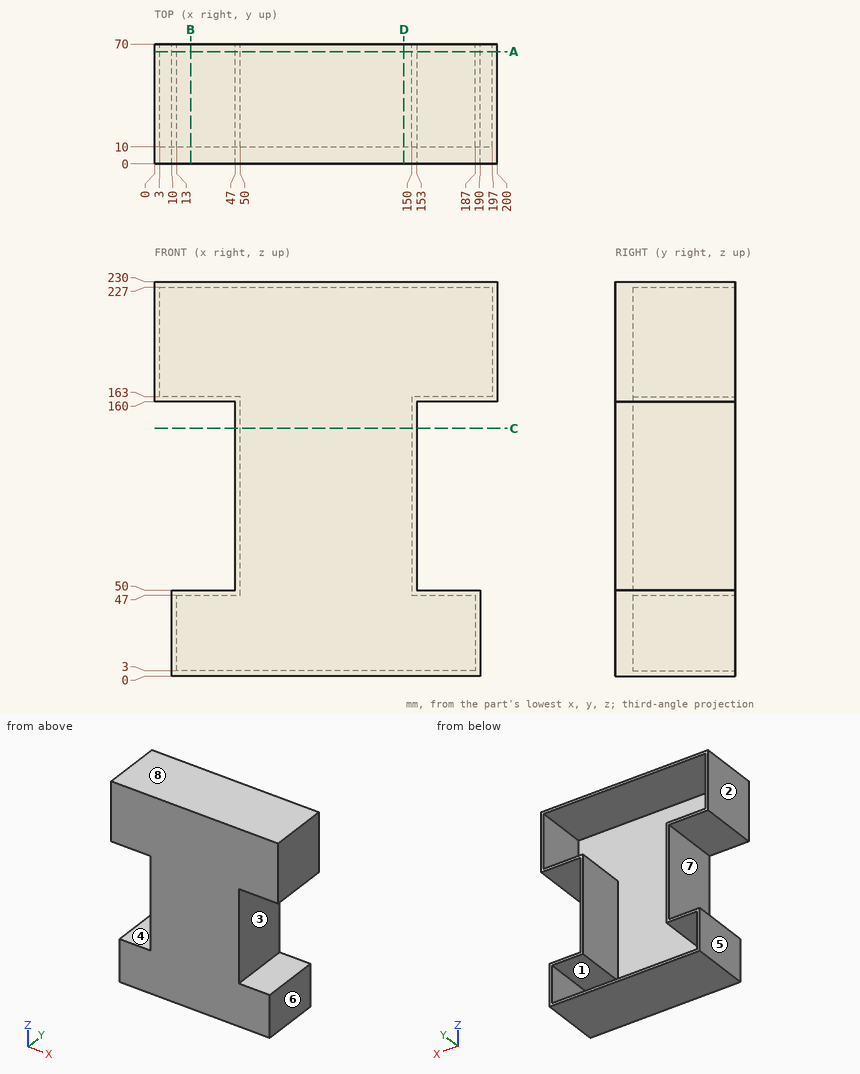
Geometry: see drawing. Coordinates: mm, zero at the bounding-box minimum. A direction names the side the tool comes from. Coordinates: 2 decimals unless noted, no trailing zeros. Loops run counter-clockwise (first coordinate to the right, second up) from the corner with the lowest first, then second, coordinate; pieces in that order, holes last. Notation, with made-up numbers: (-26.75, -22.5) - (6.25, -22.5) arc R24 cw to (6.25, -11.5) - close; hole circle Ø7 at (-7.5, 76). An arc over 180 degrees is marked (long way). Answer in a Markdown table with one row per item.
(1) Cut plane C-C on z = 144.5. Output: boundary loops of the cut face in (x, y), plus the area to 3 significant figures.
Model answer:
| item | result |
|---|---|
| outline | (47, 0) - (153, 0) - (153, 70) - (150, 70) - (150, 10) - (50, 10) - (50, 70) - (47, 70) - close |
| area | 1,420 mm² |
(2) Pin query (flat end, axial travel): P1, Ø1.5, axis at y = 41, z = 149, coming from the -X side; P2, Ø4, axis at x = 52.5, z = 33.5, coming from the +Y side; P3, Ø12, axis at y = 59, z = 34.5, coming from the +X side. Return the tip coordinate at first contact, or that it passes through.
Model answer:
| item | result |
|---|---|
| P1 | stops at x = 47 |
| P2 | stops at y = 10 |
| P3 | stops at x = 190 |
(3) Material intervals for L1, parallel to Z at x = 36, y = 66; L2, parallel to Z at x = 64, y = 55.5; L3, parallel to X at y = 18, z = 167.5, sorted ascending. Write a range as from..to.
Model answer:
| item | result |
|---|---|
| L1 | z = 0..3, 47..50, 160..163, 227..230 |
| L2 | z = 0..3, 227..230 |
| L3 | x = 0..3, 197..200 |
(4) Cut plane B-B on x = 21. Output: boundary loops of the cut face in (y, z), plus the area to 3 significant figures.
Model answer:
| item | result |
|---|---|
| outline | (0, 0) - (70, 0) - (70, 3) - (10, 3) - (10, 47) - (70, 47) - (70, 50) - (0, 50) - close; (0, 160) - (70, 160) - (70, 163) - (10, 163) - (10, 227) - (70, 227) - (70, 230) - (0, 230) - close |
| area | 1,920 mm² |
(5) Set-up query: the marked faces 1, 2, 3, 4 and 5. Return all of +Z, -Z, +X, -X, +Y, -Y with unobstructed straight access to the full face (end or side cutting, diameter ignored); none if empty.
Model answer:
| item | result |
|---|---|
| face 1 | +Y |
| face 2 | +Z, -Z, -X, +Y, -Y |
| face 3 | +X, +Y, -Y |
| face 4 | -X, +Y, -Y |
| face 5 | -Z, -X, +Y, -Y |
(6) Cut plane D-D on x = 145.5. Output: boundary loops of the cut face in (y, z).
Model answer:
| item | result |
|---|---|
| outline | (0, 0) - (70, 0) - (70, 3) - (10, 3) - (10, 227) - (70, 227) - (70, 230) - (0, 230) - close |
(7) Mould query, pull axis Z, two halves, no side actions, for the marked faces 6, 7 and 8. Classes: pulls with the +Z half, pulls with the -Z half, needs draft (parallel to the pull), parting line crosses it, or undercut.
Model answer:
| item | result |
|---|---|
| face 6 | needs draft |
| face 7 | undercut |
| face 8 | pulls with the +Z half |
(8) Cut plane A-A on y = 65.5. Output: boundary loops of the cut face in (x, z), plus the area to 3 significant figures.
Model answer:
| item | result |
|---|---|
| outline | (0, 160) - (47, 160) - (47, 50) - (10, 50) - (10, 0) - (190, 0) - (190, 50) - (153, 50) - (153, 160) - (200, 160) - (200, 230) - (0, 230) - close; hole (3, 163) - (50, 163) - (50, 47) - (13, 47) - (13, 3) - (187, 3) - (187, 47) - (150, 47) - (150, 163) - (197, 163) - (197, 227) - (3, 227) - close |
| area | 2,990 mm² |
